from build123d import *

# Parameters (mm, degrees)
SKETCH1_R                 = 11
BOSS_EXTRUDE2_DEPTH       = 4
SKETCH2_R                 = 5
BOSS_EXTRUDE3_DEPTH       = 2
SKETCH3_R                 = 11
BOSS_EXTRUDE4_DEPTH       = 1.002207304
SKETCH4_R                 = 5
BOSS_EXTRUDE5_DEPTH       = 2
SKETCH5_R                 = 11
BOSS_EXTRUDE6_DEPTH       = 1
SKETCH6_R                 = 5
BOSS_EXTRUDE7_DEPTH       = 2
SKETCH7_R                 = 11
BOSS_EXTRUDE8_DEPTH       = 1
SKETCH8_R                 = 5
BOSS_EXTRUDE9_DEPTH       = 2
BOSS_EXTRUDE10_DEPTH      = 1
BOSS_EXTRUDE10_DEPTH_BACK = 0.02884934
SKETCH9_R                 = 11
SKETCH10_R                = 5
BOSS_EXTRUDE11_DEPTH      = 2
SKETCH11_R                = 11
BOSS_EXTRUDE12_DEPTH      = 1
SKETCH12_R                = 5
BOSS_EXTRUDE13_DEPTH      = 2
SKETCH13_R                = 11
BOSS_EXTRUDE14_DEPTH      = 2
BOSS_EXTRUDE15_DEPTH      = 4
SKETCH15_W                = 10
SKETCH15_H                = 14
BOSS_EXTRUDE16_DEPTH      = 20
SKETCH17_R                = 2.5
BOSS_EXTRUDE17_DEPTH      = 3
BOSS_EXTRUDE17_TAPER      = 32
SKETCH18_R                = 0.875
CUT_EXTRUDE2_DEPTH        = 48
SKETCH19_R                = 0.2
CUT_EXTRUDE3_DEPTH        = 5
FILLET1_R                 = 2
FILLET2_R                 = 2
SKETCH20_R                = 1.25
CUT_EXTRUDE4_DEPTH        = 8
SKETCH22_R                = 1.25
CUT_EXTRUDE5_DEPTH        = 8


with BuildPart() as part:
    # Sketch1 → Boss-Extrude2 (new body)
    with BuildSketch(Plane(origin=(0, 0, 0), x_dir=(1, 0, 0), z_dir=(0, 1, 0))):
        with Locations(Location((0, 0, 0), (0, 0, 270))):
            Circle(SKETCH1_R)
    extrude(amount=-BOSS_EXTRUDE2_DEPTH)

    # Sketch2 → Boss-Extrude3 (add)
    with BuildSketch(Plane(origin=(0, -4, 0), x_dir=(-1, 0, 0), z_dir=(0, -1, 0))):
        with Locations(Location((0, 0, 0), (0, 0, 90))):
            Circle(SKETCH2_R)
    extrude(amount=BOSS_EXTRUDE3_DEPTH)

    # Sketch3 → Boss-Extrude4 (add)
    with BuildSketch(Plane.XZ.offset(6)):
        with Locations(Location((0, 0, 0), (0, 0, 90))):
            Circle(SKETCH3_R)
    extrude(amount=BOSS_EXTRUDE4_DEPTH)

    # Sketch4 → Boss-Extrude5 (add)
    with BuildSketch(Plane(origin=(0, -7.002207304, 0), x_dir=(-1, 0, 0), z_dir=(0, -1, 0))):
        with Locations(Location((0, 0, 0), (0, 0, 90))):
            Circle(SKETCH4_R)
    extrude(amount=BOSS_EXTRUDE5_DEPTH)

    # Sketch5 → Boss-Extrude6 (add)
    with BuildSketch(Plane.XZ.offset(9.002207304)):
        with Locations(Location((0, 0, 0), (0, 0, 90))):
            Circle(SKETCH5_R)
    extrude(amount=BOSS_EXTRUDE6_DEPTH)

    # Sketch6 → Boss-Extrude7 (add)
    with BuildSketch(Plane(origin=(0, -10.002207304, 0), x_dir=(-1, 0, 0), z_dir=(0, -1, 0))):
        with Locations(Location((0, 0, 0), (0, 0, 90))):
            Circle(SKETCH6_R)
    extrude(amount=BOSS_EXTRUDE7_DEPTH)

    # Sketch7 → Boss-Extrude8 (add)
    with BuildSketch(Plane(origin=(0, -12.002207304, 0), x_dir=(-1, 0, 0), z_dir=(0, -1, 0))):
        with Locations(Location((0, 0, 0), (0, 0, 270))):
            Circle(SKETCH7_R)
    extrude(amount=BOSS_EXTRUDE8_DEPTH)

    # Sketch8 → Boss-Extrude9 (add)
    with BuildSketch(Plane(origin=(0, -13.002207304, 0), x_dir=(-1, 0, 0), z_dir=(0, -1, 0))):
        with Locations(Location((0, 0, 0), (0, 0, 90))):
            Circle(SKETCH8_R)
    extrude(amount=BOSS_EXTRUDE9_DEPTH)

    # Sketch9 → Boss-Extrude10 (add, two sides: drawn at the far end of the back side and taken through both)
    with BuildSketch(Plane(origin=(0, -15.002207304, 0), x_dir=(-1, 0, 0), z_dir=(0, -1, 0)).offset(-BOSS_EXTRUDE10_DEPTH_BACK)):
        with Locations(Location((0, 0, 0), (0, 0, 270))):
            Circle(SKETCH9_R)
    extrude(amount=BOSS_EXTRUDE10_DEPTH + BOSS_EXTRUDE10_DEPTH_BACK)

    # Sketch10 → Boss-Extrude11 (add)
    with BuildSketch(Plane(origin=(0, -16.002207304, 0), x_dir=(-1, 0, 0), z_dir=(0, -1, 0))):
        with Locations(Location((0, 0, 0), (0, 0, 90))):
            Circle(SKETCH10_R)
    extrude(amount=BOSS_EXTRUDE11_DEPTH)

    # Sketch11 → Boss-Extrude12 (add)
    with BuildSketch(Plane(origin=(0, -18.002207304, 0), x_dir=(-1, 0, 0), z_dir=(0, -1, 0))):
        with Locations(Location((0, 0, 0), (0, 0, 270))):
            Circle(SKETCH11_R)
    extrude(amount=BOSS_EXTRUDE12_DEPTH)

    # Sketch12 → Boss-Extrude13 (add)
    with BuildSketch(Plane(origin=(0, -19.002207304, 0), x_dir=(-1, 0, 0), z_dir=(0, -1, 0))):
        with Locations(Location((0, 0, 0), (0, 0, 90))):
            Circle(SKETCH12_R)
    extrude(amount=BOSS_EXTRUDE13_DEPTH)

    # Sketch13 → Boss-Extrude14 (add)
    with BuildSketch(Plane(origin=(0, -21.002207304, 0), x_dir=(-1, 0, 0), z_dir=(0, -1, 0))):
        with Locations(Location((0, 0, 0), (0, 0, 270))):
            Circle(SKETCH13_R)
    extrude(amount=BOSS_EXTRUDE14_DEPTH)

    # Sketch14 → Boss-Extrude15 (add)
    with BuildSketch(Plane(origin=(0, -23.002207304, 0), x_dir=(-1, 0, 0), z_dir=(0, -1, 0))):
        with BuildLine():
            Line((5.450000001, -1.4309088), (0.900000001, -2.861817604))
            ThreePointArc((0.900000001, -2.861817604), (1e-09, -3), (-0.9, -2.861817604))
            Line((-0.9, -2.861817604), (-5.45, -1.430908802))
            ThreePointArc((-5.45, -1.430908802), (-6.5, 0), (-5.45, 1.430908802))
            Line((-5.45, 1.430908802), (-0.9, 2.861817604))
            ThreePointArc((-0.9, 2.861817604), (-1e-09, 3), (0.899999999, 2.861817605))
            Line((0.899999999, 2.861817605), (5.450000001, 1.430908804))
            ThreePointArc((5.450000001, 1.430908804), (6.5, 2e-09), (5.450000001, -1.4309088))
        make_face()
    extrude(amount=BOSS_EXTRUDE15_DEPTH)

    # Sketch15 → Boss-Extrude16 (add)
    with BuildSketch(Plane(origin=(0, -27.002207304, 0), x_dir=(-1, 0, 0), z_dir=(0, -1, 0))):
        Rectangle(SKETCH15_W, SKETCH15_H)
    extrude(amount=BOSS_EXTRUDE16_DEPTH)

    # Sketch17 → Boss-Extrude17 (add)
    with BuildSketch(Plane(origin=(0, -47.002207304, 0), x_dir=(-1, 0, 0), z_dir=(0, -1, 0))):
        Circle(SKETCH17_R)
    extrude(amount=BOSS_EXTRUDE17_DEPTH, taper=BOSS_EXTRUDE17_TAPER)

    # Sketch18 → Cut-Extrude2 (cut)
    with BuildSketch(Plane(origin=(0, 0, 0), x_dir=(1, 0, 0), z_dir=(0, 1, 0))):
        with Locations(Location((0, 0, 0), (0, 0, 270))):
            Circle(SKETCH18_R)
    extrude(amount=-CUT_EXTRUDE2_DEPTH, mode=Mode.SUBTRACT)

    # Sketch19 → Cut-Extrude3 (cut)
    with BuildSketch(Plane(origin=(0, -50.002207304, 0), x_dir=(-1, 0, 0), z_dir=(0, -1, 0))):
        with Locations(Location((0, 0, 0), (0, 0, 90))):
            Circle(SKETCH19_R)
    extrude(amount=-CUT_EXTRUDE3_DEPTH, mode=Mode.SUBTRACT)

    # Fillet1
    fillet1_edges = [part.edges().sort_by_distance(p)[0] for p in [
        (5, -27.002207304, -4.286213628),
        (5, -27.002207304, 4.286213628),
        (5, -37.002207304, -7),
        (0, -27.002207304, 7),
        (5, -37.002207304, 7),
        (-5, -27.002207304, 4.286213627),
        (-5, -27.002207304, -4.286213629),
        (0, -27.002207304, -7),
        (-5, -37.002207304, -7),
        (5, -47.002207304, 0),
        (0, -47.002207304, 7),
        (-5, -47.002207304, 0),
        (0, -47.002207304, -7),
    ]]
    fillet(fillet1_edges, radius=FILLET1_R)

    # Fillet2
    # the kernel refuses this fillet: 2 mm, written as the material it takes off along each edge
    with BuildSketch(Plane(origin=(-3, -29.002207304, 5), x_dir=(0, 0, 1), z_dir=(-1, 0, 0))) as fillet2_piece_1_section:
        Polygon((0, 0), (FILLET2_R, 0), (FILLET2_R, FILLET2_R), (0, FILLET2_R), align=None)
    fillet2_piece_1 = extrude(amount=FILLET2_R, mode=Mode.PRIVATE)
    fillet2_piece_1 = fillet2_piece_1 - Plane(origin=(-3, -29.002207304, 5), x_dir=(0, -0.7071067811865475, -0.7071067811865475), z_dir=(-1, 0, 0)) * Sphere(FILLET2_R, mode=Mode.PRIVATE)
    add(fillet2_piece_1, mode=Mode.SUBTRACT)
    with BuildSketch(Plane(origin=(-3, -45.002207304, 5), x_dir=(0, 0, 1), z_dir=(-1, 0, 0))) as fillet2_piece_2_section:
        Polygon((0, 0), (FILLET2_R, 0), (FILLET2_R, -FILLET2_R), (0, -FILLET2_R), align=None)
    fillet2_piece_2 = extrude(amount=FILLET2_R, mode=Mode.PRIVATE)
    fillet2_piece_2 = fillet2_piece_2 - Plane(origin=(-3, -45.002207304, 5), x_dir=(0, 0.7071067811865475, -0.7071067811865475), z_dir=(-1, 0, 0)) * Sphere(FILLET2_R, mode=Mode.PRIVATE)
    add(fillet2_piece_2, mode=Mode.SUBTRACT)
    with BuildSketch(Plane(origin=(-5, -29.002207304, 7), x_dir=(0, 0, -1), z_dir=(0, -1, 0))) as fillet2_piece_3:
        with BuildLine():
            CenterArc((FILLET2_R, FILLET2_R), FILLET2_R, 180, 90)
            Line((0, FILLET2_R), (0, 0))
            Line((0, 0), (FILLET2_R, 0))
        make_face()
    extrude(amount=16, mode=Mode.SUBTRACT)

    # Sketch20 → Cut-Extrude4 (cut)
    with BuildSketch(Plane(origin=(0, 0, 0), x_dir=(1, 0, 0), z_dir=(0, 1, 0))):
        with Locations(Location((-5.5, 5.5, 0), (0, 0, 90))):
            Circle(SKETCH20_R)
        with Locations(Location((5.5, 5.5, 0), (0, 0, 90))):
            Circle(SKETCH20_R)
        with Locations(Location((-5.5, -5.5, 0), (0, 0, 90))):
            Circle(SKETCH20_R)
        with Locations(Location((5.5, -5.5, 0), (0, 0, 90))):
            Circle(SKETCH20_R)
    extrude(amount=-CUT_EXTRUDE4_DEPTH, mode=Mode.SUBTRACT)

    # Sketch22 → Cut-Extrude5 (cut)
    with BuildSketch(Plane(origin=(0, 0, 0), x_dir=(1, 0, 0), z_dir=(0, 1, 0))):
        with Locations(Location((-8.5, 0, 0), (0, 0, 90))):
            Circle(SKETCH22_R)
        with Locations(Location((8.5, 0, 0), (0, 0, 90))):
            Circle(SKETCH22_R)
    extrude(amount=-CUT_EXTRUDE5_DEPTH, mode=Mode.SUBTRACT)


solid = part.part
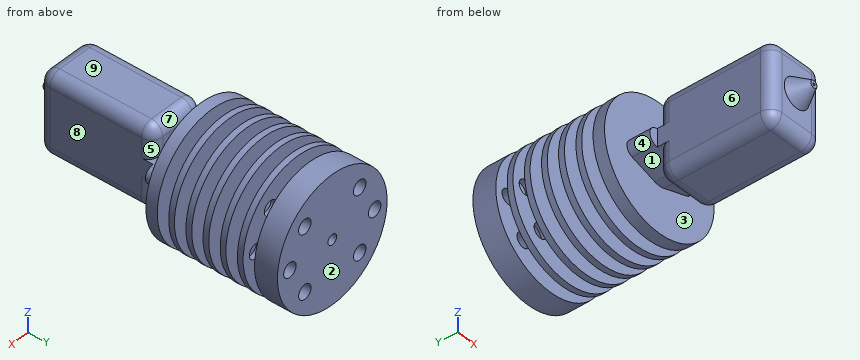
Source: CAD feature listing. Evaluate the final solid. Frame: model axes, mm. Face numbers are marked on the shaded views. A direction names the side the tool comes from. Coordinates: 2 decimals unless noted, no trailing zeros. Order: outer loops, then holes, each group sorted by start corner. A loop starts at its lowest first (then second) coordinate and runs counter-clockwise, first axis right, second up. Notation, with made-up numbers: M -2,66.5 L 19,66.5 A28 ccw 19,91.5 Z; hole C -27.5,-25.75 d8. An arc over 180 degrees is marked long. Write each question's results on one line, items separated by ' | '. Start each with the question number.
1. Pin query (flat end, axial travel): pin 1 (12 mm diameter, centred on x = 6, z = -6.5, fed in from -Y); pin 2 (3 mm diameter, centred on y = -41.5, z = 0.5, fed in from -X); pin 3 (10 mm diameter, centred on x = -4.5, y = -41, fed in from -Z). Return the tip coordinate at first contact, or that it passes through.
2. Section D-D, the plane y = -8. Return the cut outline in (x, z) (3 decimals).
3. Material intervals for L1, parallel to X at y = -6.7, z = 0 (3 decimals); L2, parallel to Y at x = -6.5, z = 5; L3, parallel to X at y = -1.6, z = -5.5, sorted ascending.
4. Reachability of the marked faces 5, 6, 7, 8 and 9 from +Z, -Z, +X, -X, +Y, -Y: full face, straight path, thin tool, end or side. Return the list, or none.
5. Section A-A, the plane y = -26. Return the cut outline in (x, z) (3 decimals).
6. Section B-B, the plane z = 5.5. State how many separate pieces and enclosed holes the cut face has, then the cut area to 3 significant figures.
7. Draft query along Y for the marked faces 1, 2, 3 and 4. Return one class per face: +Y half, -Y half, draft (parallel to the pull), parting line (faces both ways), or undercut.
Solution:
1) pin 1: y = -47 | pin 2: x = -5 | pin 3: z = -7
2) outline: C 0,0 d10; hole C 0,0 d1.75
3) L1: -11 to -9.75, -7.25 to -0.875, 0.875 to 7.25, 9.75 to 11 | L2: -23 to -21, -19 to -18, -16 to -14.97, -13 to -12, -10 to -9 | L3: -9.53 to -6.75, -4.25 to 4.25, 6.75 to 9.53
4) face 5: +Z, +X | face 6: +Z, -Z, -X, -Y | face 7: +Z, +X, -X | face 8: +Z, -Z, +X, -Y | face 9: +Z, +X, -X, -Y
5) outline: M -5.45,-1.431 L -0.9,-2.862 A3 ccw 0.9,-2.862 L 5.45,-1.431 A1.5 ccw 5.45,1.431 L 0.9,2.862 A3 ccw -0.9,2.862 L -5.45,1.431 A1.5 ccw Z; hole C 0,0 d1.75
6) separate pieces: 12 | enclosed holes: 0 | area: 378 mm²
7) face 1: undercut | face 2: +Y half | face 3: undercut | face 4: draft
